Part model, mm, in its own coordinate system. A direction names the side the tool comes from. Coordinates: 2 decimals unless noted, no trailing zeros. Loops run counter-clockwise (first coordinate to the right, second up) from the corner with the lowest first, then second, coordinate; pieces in that order, holes last. Notation, with made-up numbers: (63.5, 13.25) - (90.5, 13.25) arc R34 ccw to (90.5, 50.25) - close; hole circle Ø5 at (10, -2.5). An arc over 180 degrees is marked (long way). Answer as CSV lines item,"result".
from build123d import *

# Parameters (mm, degrees)
BOSS_EXTRUDE1_DEPTH         = 29.5
CHAMFER1_SIZE               = 1
SKETCH4_W                   = 10.79057785
SKETCH4_H                   = 9.5
HOLE_WIZARD_M51_D           = 5.3
HOLE_WIZARD_M51_CSINK_D     = 10.4
HOLE_WIZARD_M51_CSINK_ANGLE = 90


with BuildPart() as part:
    # Sketch2 → Boss-Extrude1 (new body)
    with BuildSketch(Plane.XY):
        with BuildLine():
            Line((11.958260743, 1), (25, 1))
            Line((25, 1), (25, 19))
            Line((25, 19), (-25, 19))
            Line((-25, 19), (-25, 1))
            Line((-25, 1), (-11.958260743, 1))
            ThreePointArc((-11.958260743, 1), (0, 12), (11.958260743, 1))
        make_face()
    extrude(amount=BOSS_EXTRUDE1_DEPTH)

    # Chamfer1
    chamfer1_edges = [part.edges().sort_by_distance(p)[0] for p in [
        (-25, 19, 14.75),
        (25, 19, 14.75),
        (25, 1, 14.75),
        (-25, 1, 14.75),
    ]]
    chamfer(chamfer1_edges, length=CHAMFER1_SIZE)

    # Sketch4 → Cut-Revolve1 (revolve, cut)
    with BuildSketch(Plane(origin=(0, 0, 0), x_dir=(-1, 0, 0), z_dir=(0, -1, 0))):
        with Locations((9.604711075, -14.75)):
            Rectangle(SKETCH4_W, SKETCH4_H)
    revolve(axis=Axis((0, 0, 0), (0, 0, 1)), mode=Mode.SUBTRACT)

    # Зенковка для  винта с плоской головкой M51 (through all)
    with Locations(Plane(origin=(0, 19, 0), x_dir=(1, 0, 0), z_dir=(0, 1, 0))):
        with Locations((-20, -14.75), (20, -14.75)):
            CounterSinkHole(HOLE_WIZARD_M51_D / 2, HOLE_WIZARD_M51_CSINK_D / 2, counter_sink_angle=HOLE_WIZARD_M51_CSINK_ANGLE)


solid = part.part
Q1. Two-plate mould, pull along Z, no slides. Class faces 1 (the face through (-17.23, 16.57, 14.63)), 2 (the face through (25, 10, 15)), 3 (the face through (0, 14, 0)): released by +Z, released by -Z, zero draft, split by the parting line, or undercut.
Results:
face 1,"undercut"
face 2,"zero draft"
face 3,"released by -Z"
Q2. Flat gauge pin, fed straight in: pin 1 (7 mm diameter, centred on x = 20, z = 14.75, fed in from +Y). Where does the tip first touch, or does it go through?
Results:
pin 1,"stops at y = 17.3"
Q3. Saw through at B-B (z = 14.75). Give the cut face in (x, y).
Results:
outline,"(-25, 2) - (-24, 1) - (-22.65, 1) - (-22.65, 16.45) - (-24.6, 18.4) - (-25, 18) - close; (-17.35, 1) - (-14.97, 1) arc R15 cw to (14.97, 1) - (17.35, 1) - (17.35, 16.45) - (14.8, 19) - (-14.8, 19) - (-17.35, 16.45) - close; (22.65, 1) - (24, 1) - (25, 2) - (25, 18) - (24.6, 18.4) - (22.65, 16.45) - close"
Q4. Which spindle directions (+Z, -Z, +X, -X, +Y, -Y) get a long thin tool onto all of the face, cutting with end or side? Do faces 4 (the face through (2, 12, 19.5)), 5 (the face through (24.5, 1.5, 14.5)). Say none if no direction does.
Results:
face 4,"-Y"
face 5,"+Z, -Z, +X, -Y"
Q5. Saw through at A-A (x = -20). Give the cut face in (y, z).
Results:
outline,"(1, 0) - (19, 0) - (19, 9.55) - (16.45, 12.1) - (1, 12.1) - close; (1, 17.4) - (16.45, 17.4) - (19, 19.95) - (19, 29.5) - (1, 29.5) - close"
Q6. Saw through at D-D (x = 0). Give the cut face in (y, z).
Results:
outline,"(12, 0) - (19, 0) - (19, 29.5) - (12, 29.5) - (12, 19.5) - (15, 19.5) - (15, 10) - (12, 10) - close"
Q7. Saw through at C-C (y = 4.25). Give the cut face in (x, z).
Results:
outline,"(-25, 0) - (-11.22, 0) - (-11.22, 10) - (-14.39, 10) - (-14.39, 19.5) - (-11.22, 19.5) - (-11.22, 29.5) - (-25, 29.5) - close; (11.22, 0) - (25, 0) - (25, 29.5) - (11.22, 29.5) - (11.22, 19.5) - (14.39, 19.5) - (14.39, 10) - (11.22, 10) - close; hole circle Ø5.3 at (-20, 14.75); hole circle Ø5.3 at (20, 14.75)"
Q8. Wall check: L1, parallel to Z at x = 6, y = 12.5; L2, parallel to Z at x = 20, y = 13; L3, parallel to X at y = 8, z = 14.75. Give the ranges that are in metal, low to high.
Results:
L1,"z = 0 to 10, 19.5 to 29.5"
L2,"z = 0 to 12.1, 17.4 to 29.5"
L3,"x = -25 to -22.65, -17.35 to -12.69, 12.69 to 17.35, 22.65 to 25"
